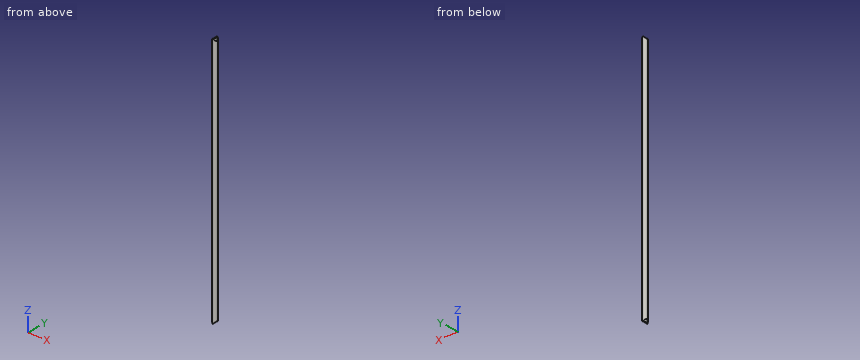
Autodesk Inventor part; units mm, degrees
ref_plane "Start plane" through (0, 0, 0) normal (0, 0, 1) x (1, 0, 0)
ref_plane "End plane" through (0, 0, 2143.252) normal (0, 0, 1) x (1, 0, 0)
ref_plane "Work Plane4" through (-457.2, 0, 0) normal (1, 0, 0) x (0, 0, -1)
ref_plane "Start plane" through (0, 0, 0) normal (0, 0, 1) x (1, 0, 0)
ref_plane "End plane" through (0, 0, 2143.252) normal (0, 0, 1) x (1, 0, 0)
sketch "Sketch" plane through (0, 0, 0) normal (0, 0, 1) x (1, 0, 0)
  circle A0 centre (0, 0) radius 17.526
  circle A1 centre (0, 0) radius 21.082
  dimension "d0" = 42.164
  dimension "d1" = 3.556
extrude "Body" add sketch "Sketch" along normal up to surface (2143.252 mm away) from surface at 0
sketch "Sketch3" plane through (0, 0, 0) normal (0, 0, 1) x (1, 0, 0)
  line L0 (0, 0) -> (10, 0)
ref_plane "Work Plane3" through (0, 0, 0) normal (0, -1, 0) x (1, 0, 0)
sketch "Sketch4" plane through (0, 0, 0) normal (0, -1, 0) x (1, 0, 0)
  line L0 (-2, 0) -> (12, 0)
  line L1 (-2, 2143.252) -> (12, 2143.252)
  dimension "d7" = 2143.252
ref_plane "Work Plane4" through (-457.2, 0, 0) normal (1, 0, 0) x (0, 0, -1)
ref_plane "Work Plane5" through (50.8, 0, 0) normal (1, 0, 0) x (0, 0, -1)
ref_plane "Work Plane6" through (-203.2, 0, 0) normal (1, 0, 0) x (0, 0, -1)
sketch "Sketch5" plane through (-203.2, 0, 0) normal (1, 0, 0) x (0, 0, -1)
  circle A0 centre (0, 0) radius 21.082
  circle A1 centre (0, 0) radius 17.526
extrude "Extrusion2" cut sketch "Sketch5" along normal up to surface (508 mm away) from surface at -254 contours A0 | A1
ref_plane "Work Plane7" through (50.8, 0, 2143.252) normal (-1, 0, 0) x (0, 0, 1)
ref_plane "Work Plane8" through (-457.2, 0, 2143.252) normal (-1, 0, 0) x (0, 0, 1)
ref_plane "Work Plane9" through (-203.2, 0, 2143.252) normal (-1, 0, 0) x (0, 0, 1)
sketch "Sketch6" plane through (-203.2, 0, 2143.252) normal (-1, 0, 0) x (0, 0, 1)
  circle A0 centre (0, 0) radius 21.082
  circle A1 centre (0, 0) radius 17.526
extrude "Extrusion3" cut sketch "Sketch6" along normal up to surface (508 mm away) from surface at -254 contours A0 | A1
ref_plane "Work Plane10" through (0, 21.082, 2143.252) normal (0, 0, 1) x (0, -1, 0)
equation "\"d0\" = G_H"
equation "\"d1\" = G_T"
equation "\"d2\" = G_L"
equation "\"G_H\" = 42.164"
equation "\"G_T\" = 3.556"
equation "\"G_L\" = d7"
equation "\"G_OFFSET_START\" = 0"
equation "\"G_OFFSET_END\" = 0"
equation "\"d5\" = G_OFFSET_END + B_L"
equation "\"B_L\" = 2143.252"
properties part number "ANSI - 1 1/4 x 0.140 - 84.38" material "Aluminum 6061"
Can you work these out from the model? Positions are in its coordinate system, mm. Coordinates: 2 decimals unless noted, no trailing zeros. Loops run counter-clockwise (first coordinate to the right, second up) from the corner with the lowest first, then second, coordinate; pieces in that order, holes last. Notation, with made-up numbers: (67.25, -26.75) - (124.25, -26.75) arc R22 ccw to (124.25, -7.75) - close; hole circle Ø10 at (59.25, 78.25). An arc over 180 degrees is marked (long way). Answer as a JSON object with one key per item and string values. Group by question number.
Item 1: For pin 1 (3 mm diameter, centred on x = -8, z = 957, fed in from +Y); pin 2 (4 mm diameter, centred on x = 3, z = 1879.5, fed in from -Y); pin 3 (8 mm diameter, centred on y = -7.5, z = 1426.5, fed in from -X); pin 4 (6 mm diameter, centred on x = -4.5, y = 11.5, fed in from -Z), each with a flat end and sliding along its axis, tell me the tip position at first contact or that it passes through.
Item 2: If we section it at A-A (y = 0): List the corners of the cut face in (x, z) for me, plus the area to 3 significant figures.
Item 3: If we section it at C-C (z = 819): List the corners of the cut face in (x, y) for me, plus the area to 3 significant figures.
Item 4: If we section it at B-B (x = 0): List the corners of the cut face in (y, z) for me.
Item 5: If I drill on L1, parallel to Y at x = 0, z = 1082; L2, parallel to X at y = -1.5, z = 339, over which ranges is the centre line in solid material (lowest first)? Write a range as from..to.
Returned:
{
 "1": {"pin 1": "stops at y = 20.05", "pin 2": "stops at y = -21.06", "pin 3": "stops at x = -20.79", "pin 4": "passes through"},
 "2": {"outline": "(-21.08, 21.08) - (-17.53, 21.08) - (-17.53, 2122.17) - (-21.08, 2122.17) - close; (17.53, 21.08) - (21.08, 21.08) - (21.08, 2122.17) - (17.53, 2122.17) - close", "area": "14,900 mm²"},
 "3": {"outline": "circle Ø42.16 at (0, 0); hole circle Ø35.05 at (0, 0)", "area": "431 mm²"},
 "4": {"outline": "(-21.08, 0) arc R21.08 cw to (-17.53, 11.72) - (-17.53, 2131.53) arc R21.08 cw to (-21.08, 2143.25) - close; (17.53, 11.72) arc R21.08 cw to (21.08, 0) - (21.08, 2143.25) arc R21.08 cw to (17.53, 2131.53) - close"},
 "5": {"L1": "y = -21.08..-17.53, 17.53..21.08", "L2": "x = -21.03..-17.46, 17.46..21.03"}
}
